from build123d import *

# Parameters (mm, degrees)
CROQUIS1_R              = 9.5
SALIENTE_EXTRUIR1_DEPTH = 12
CROQUIS2_R              = 6
SALIENTE_EXTRUIR2_DEPTH = 30
CHAFL_N1_SIZE           = 1
CORTAR_EXTRUIR1_DEPTH   = 8


with BuildPart() as part:
    # Croquis1 → Saliente-Extruir1 (new body)
    with BuildSketch(Plane.XY):
        Circle(CROQUIS1_R)
    extrude(amount=SALIENTE_EXTRUIR1_DEPTH)

    # Croquis2 → Saliente-Extruir2 (add)
    with BuildSketch(Plane(origin=(0, 0, 0), x_dir=(-1, 0, 0), z_dir=(0, 0, -1))):
        with Locations(Location((0, 0, 0), (0, 0, 180))):
            Circle(CROQUIS2_R)
    extrude(amount=SALIENTE_EXTRUIR2_DEPTH)

    # Chaflán1
    chafl_n1_edges = [part.edges().sort_by_distance(p)[0] for p in [
        (-9.5, 0, 12),
        (-6, 0, -30),
    ]]
    chamfer(chafl_n1_edges, length=CHAFL_N1_SIZE)

    # Croquis3 → Cortar-Extruir1 (cut)
    with BuildSketch(Plane.XY.offset(12)):
        Polygon((5.8, 0), (2.9, 5.022947342), (-2.9, 5.022947342), (-5.8, 0), (-2.9, -5.022947342), (2.9, -5.022947342), align=None)
    extrude(amount=-CORTAR_EXTRUIR1_DEPTH, mode=Mode.SUBTRACT)


solid = part.part
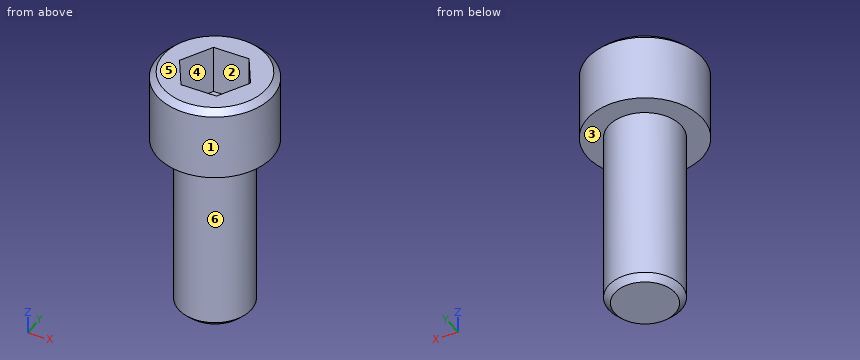
Work out the finished part from the listing and answer in its coordinate system (mm). Face numbers are marked on the shaded views. A direction names the side the tool comes from. Round coordinates to 2 decimals unless told otherwise and drop trailing zeros. Order: outer loops, then holes, each group sorted by start corner. A loop starts at its lowest first (then second) coordinate and runs counter-clockwise, first axis right, second up. Notation, with made-up numbers: M 72.25,-19 L 103.25,-19 A19 ccw 103.25,0 Z; hole C 16,-14.75 d4. An arc over 180 degrees is marked long. Put each result on its own line as item: value. Start each with the question number.
Q1. Section C-C, the plane z = -15 is taken. Write down the section's boundary in (x, y).
Q2. For a pull along Y with two mould halves and no side action, classify the marked faces 1, 2 and 3 as pulls with the +Y half, pulls with the -Y half, needs draft (parallel to the pull), parting line crosses it, or undercut.
Q3. Flat-ended cylindrical pins translate along their axes: pin 1 (4 mm diameter, centred on x = -3, z = -10.5, fed in from -Y); pin 2 (6.5 mm diameter, centred on x = 1.5, z = 10, fed in from +Y); pin 3 (1.5 mm diameter, centred on x = 7, z = -1.5, fed in from +Y); pin 4 (5 mm diameter, centred on x = 0.5, z = -4.5, fed in from +Y). Find the tip coordinate at first contact, or state that the pin passes through.
Q4. Section A-A, the plane x = 0 is taken. Write down the section's boundary in (y, z).
Q5. Straight lines are drawn through the part: L1, parallel to Z at x = -4.5, y = 5; L2, parallel to Z at x = 1, y = 0.5; L3, parallel to X at y = 1.5, z = -10. For each, find the intervals that lie inside material, in ascending order. Write a range as [from, to].
Q6. Section B-B, the plane z = 1 is taken. Write down the section's boundary in (x, y).
Q7. A tool of negligible diameter and unlimited length cuts with its end or side. For the marked faces 4, 5 and 6, from which of +Z, -Z, +X, -X, +Y, -Y can it reach the whole face along a straight path? Write none if from no direction.
Findings below:
1. outline: C 0,0 d12
2. face 1: parting line crosses it
2. face 2: undercut
2. face 3: needs draft
3. pin 1: stops at y = -5.92
3. pin 2: stops at y = 9.5
3. pin 3: passes through
3. pin 4: stops at y = 6
4. outline: M -9.5,0 L -6,0 L -6,-29 L -5,-30 L 5,-30 L 6,-29 L 6,0 L 9.5,0 L 9.5,11 L 8.5,12 L 5.02,12 L 5.02,4 L -5.02,4 L -5.02,12 L -8.5,12 L -9.5,11 Z
5. L1: z = [0, 12]
5. L2: z = [-30, 4]
5. L3: x = [-5.81, 5.81]
6. outline: C 0,0 d19
7. face 4: +Z
7. face 5: +Z, +X, -X, +Y, -Y
7. face 6: -Z
